from build123d import *

# Parameters (mm, degrees)
SKETCH1_W           = 900
SKETCH1_H           = 30
BOSS_EXTRUDE1_DEPTH = 30
SKETCH2_W           = 15
SKETCH2_H           = 100
BOSS_EXTRUDE2_DEPTH = 30
SKETCH3_W           = 15
SKETCH3_H           = 15
BOSS_EXTRUDE3_DEPTH = 15
SKETCH4_W           = 177.04771777
SKETCH4_H           = 15
BOSS_EXTRUDE4_DEPTH = 20


with BuildPart() as part:
    # Sketch1 → Boss-Extrude1 (new body)
    with BuildSketch(Plane(origin=(0, 0, 0), x_dir=(1, 0, 0), z_dir=(0, 1, 0))):
        Rectangle(SKETCH1_W, SKETCH1_H)
    extrude(amount=BOSS_EXTRUDE1_DEPTH)

    # Sketch2 → Boss-Extrude2 (add)
    with BuildSketch(Plane(origin=(0, 30, 0), x_dir=(1, 0, 0), z_dir=(0, 1, 0))):
        Polygon((-450, 15), (-603.496801426, -85), (-426.449083656, -85), (-426.449083656, 15), align=None)
        with Locations((442.5, -35)):
            Rectangle(SKETCH2_W, SKETCH2_H)
    extrude(amount=-BOSS_EXTRUDE2_DEPTH)

    # Sketch3 → Boss-Extrude3 (add)
    with BuildSketch(Plane(origin=(0, 30, 0), x_dir=(1, 0, 0), z_dir=(0, 1, 0))):
        Polygon((-603.496801426, -85), (-580.472281212, -70), (-426.449083656, -70), (-426.449083656, -85), align=None)
        with Locations((442.5, -77.5)):
            Rectangle(SKETCH3_W, SKETCH3_H)
    extrude(amount=BOSS_EXTRUDE3_DEPTH)

    # Sketch4 → Boss-Extrude4 (add)
    with BuildSketch(Plane.XY.offset(85)):
        with Locations((-514.972942541, 37.5)):
            Rectangle(SKETCH4_W, SKETCH4_H)
        Polygon((435, 45), (450, 45), (450, 30), (435, 29.894509732), align=None)
    extrude(amount=BOSS_EXTRUDE4_DEPTH)

    # Mirror1: part across plane


with BuildPart() as part_1:
    add(part.part)
    add(part.part.mirror(Plane(origin=(450, 30, -15), x_dir=(0, 0, 1), z_dir=(-1, 0, 0))))


solid = part_1.part
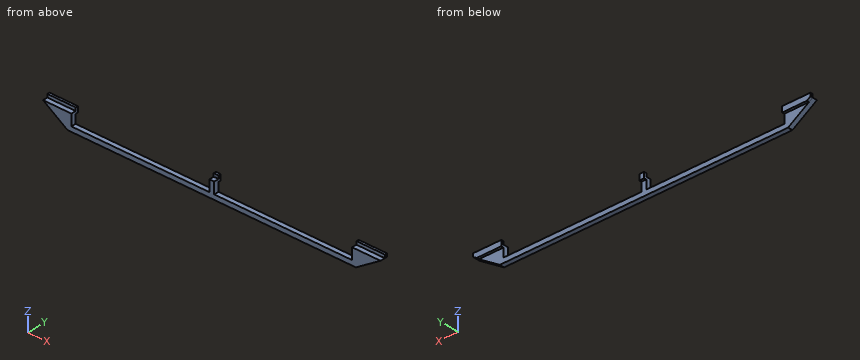
The listing builds one solid part. Answer for the finished solid, in the listing's coordinates (mm). Coordinates: 2 decimals unless noted, no trailing zeros. Write each loop counter-clockwise with the first axis right and the second up, starting at its lowest first coordinate (ties: lowest second). Pieces come first, ordered by that corner, then holes. Notation, with made-up numbers: (61.5, 35) - (97.5, 35) arc R25 cw to (97.5, 66) - close; hole circle Ø9 at (-38.5, 42). An arc over 180 degrees is marked (long way). Put each result on its own line as item: value.
1. The part is cut by section B-B on y = 22. Give the vertices of the cut face in (x, z), plus the area to 3 significant figures.
Answer sheet:
outline: (-603.5, 85) - (-450, -15) - (1350, -15) - (1503.5, 85) - (1326.45, 85) - (1326.45, 15) - (465, 15) - (465, 85) - (435, 85) - (435, 15) - (-426.45, 15) - (-426.45, 85) - close
area: 74,700 mm^2
2. The part is cut by section A-A on z = 50. Give the vertices of the cut face in (x, y).
Answer sheet:
outline: (-549.77, 0) - (-426.45, 0) - (-426.45, 30) - (-549.77, 30) - close; (435, 0) - (465, 0) - (465, 30) - (435, 30) - close; (1326.45, 0) - (1449.77, 0) - (1449.77, 30) - (1326.45, 30) - close
3. The part is cut by section C-C on x = -473.5. Give the vertices of the cut face in (y, z).
Answer sheet:
outline: (0, 0.31) - (30, 0.31) - (30, 70) - (45, 70) - (45, 105) - (30, 105) - (30, 85) - (0, 85) - close
4. Flat-ended cylindrical pins translate along their axes: pin 1 Ø2 at (y, z) = (10, 46.5) entering from +X; pin 2 Ø24 at (x, y) = (701.5, 12.5) entering from +Z; pin 3 Ø2 at (x, z) = (926.5, 11) entering from -Y; pin 4 Ø8 at (y, z) = (22.5, 72) entering from +X. Find the tip coordinate at first contact, or state that the pin passes through.
Answer sheet:
pin 1: stops at x = 1445.94
pin 2: stops at z = 15
pin 3: stops at y = 0
pin 4: stops at x = 1489.68
5. The part is cut by section D-D on x = 1106. Give the vertices of the cut face in (y, z), plus the area to 3 significant figures.
Answer sheet:
outline: (0, -15) - (30, -15) - (30, 15) - (0, 15) - close
area: 900 mm^2
6. Find the intervals of material crossed by line 1 along X through (y, z) = (36, 86); line 2 along X through (y, z) = (3.5, 18.5); line 3 along Z through (x, y) = (442, 33), in increasing order. Write a range as from..to.
Answer sheet:
line 1: x = -603.5..-426.45, 435..465, 1326.45..1503.5
line 2: x = -501.42..-426.45, 435..465, 1326.45..1401.42
line 3: z = 70..105
